```python
from build123d import *

# Parameters (mm, degrees)
BOSS_EXTRUDE1_DEPTH      = 20
SKETCH2_R                = 26.722222222
SKETCH2_R_2              = 17.722222222
BOSS_EXTRUDE2_DEPTH      = 20
CUT_EXTRUDE1_DEPTH       = 65
SKETCH4_R                = 15
BOSS_EXTRUDE3_DEPTH      = 65
CIRPATTERN1_COUNT        = 4
SKETCH5_W                = 98.755733185
SKETCH5_H                = 100
CUT_EXTRUDE2_DEPTH       = 216.315330002
CUT_EXTRUDE2_DEPTH_BACK  = 216.315330002
MOVE_FACE1_BY            = 9
SKETCH6_R                = 26.722222222
SKETCH6_R_2              = 17.722222222
BOSS_EXTRUDE4_DEPTH      = 5
BOSS_EXTRUDE4_DEPTH_BACK = 45


with BuildPart() as part:
    # Sketch1 → Boss-Extrude1 (new, symmetric)
    with BuildSketch(Plane.XY):
        with BuildLine():
            Line((-140.311288741, 0), (-45, 0))
            ThreePointArc((-45, 0), (-43.812144397, 10.271124735), (-40.311288741, 20))
            Line((-40.311288741, 20), (-140.311288741, 20))
            Line((-140.311288741, 20), (-140.311288741, 0))
        make_face()
        with BuildLine():
            ThreePointArc((-40.311288741, -20), (-43.812144397, -10.271124735), (-45, 0))
            Line((-45, 0), (-140.311288741, 0))
            Line((-140.311288741, 0), (-140.311288741, -20))
            Line((-140.311288741, -20), (-40.311288741, -20))
        make_face()
        with BuildLine():
            ThreePointArc((-25, 0), (-17.67766953, 17.67766953), (0, 25))
            Line((0, 25), (9, 25))
            Line((9, 25), (9, 45))
            Line((9, 45), (0, 45))
            ThreePointArc((0, 45), (-23.717082451, 38.242646352), (-40.311288741, 20))
            ThreePointArc((-40.311288741, 20), (-43.812144397, 10.271124735), (-45, 0))
            Line((-45, 0), (-25, 0))
        make_face()
        with BuildLine():
            ThreePointArc((0, -25), (-17.67766953, -17.67766953), (-25, 0))
            Line((-25, 0), (-45, 0))
            ThreePointArc((-45, 0), (-43.812144397, -10.271124735), (-40.311288741, -20))
            ThreePointArc((-40.311288741, -20), (-23.717082451, -38.242646352), (0, -45))
            Line((0, -45), (9, -45))
            Line((9, -45), (9, -25))
            Line((9, -25), (0, -25))
        make_face()
    extrude(amount=BOSS_EXTRUDE1_DEPTH, both=True)

    # Sketch2 → Boss-Extrude2 (add)
    with BuildSketch(Plane(origin=(0, 45, 0), x_dir=(1, 0, 0), z_dir=(0, 1, 0))):
        with Locations((26.722222222, 0)):
            Circle(SKETCH2_R)
        with Locations(Location((26.722222222, 0, 0), (0, 0, 270))):
            Circle(SKETCH2_R_2, mode=Mode.SUBTRACT)
    boss_extrude2 = extrude(amount=-BOSS_EXTRUDE2_DEPTH)

    # Mirror1: Boss-Extrude2 across plane
    add(boss_extrude2.mirror(Plane.ZX))

    # Sketch3 → Cut-Extrude1 (cut)
    with BuildSketch(Plane.ZY.offset(140.311288741)):
        Polygon((-12.5, 20), (-20, 20), (-20, 12.5), align=None)
    cut_extrude1 = extrude(amount=-CUT_EXTRUDE1_DEPTH, mode=Mode.SUBTRACT)

    # Sketch4 → Boss-Extrude3 (add)
    with BuildSketch(Plane.ZY.offset(140.311288741)):
        with Locations(Location((0, 0, 0), (0, 0, 180))):
            Circle(SKETCH4_R)
    extrude(amount=BOSS_EXTRUDE3_DEPTH)

    # CirPattern1: Cut-Extrude1 ×4 about axis
    cirpattern1_axis = Axis((0, 0, 0), (1, 0, 0))
    for i in range(1, CIRPATTERN1_COUNT):
        add(cut_extrude1.rotate(cirpattern1_axis, i * 360 / CIRPATTERN1_COUNT), mode=Mode.SUBTRACT)

    # Sketch5 → Cut-Extrude2 (cut, two sides)
    with BuildSketch(Plane.XY.offset(20)) as cut_extrude2_sk:
        with Locations((9.066577851, 0)):
            Rectangle(SKETCH5_W, SKETCH5_H)
    extrude(amount=CUT_EXTRUDE2_DEPTH, mode=Mode.SUBTRACT)
    extrude(cut_extrude2_sk.sketch, amount=-CUT_EXTRUDE2_DEPTH_BACK, mode=Mode.SUBTRACT)

    # Move Face1: a face moved outward by 9.0
    extrude(part.faces().sort_by_distance((-40.311288741, 0, 0))[0], amount=MOVE_FACE1_BY, dir=(1, 0, 0))

    # Sketch6 → Boss-Extrude4 (add, two sides)
    with BuildSketch(Plane(origin=(0, 20, 0), x_dir=(1, 0, 0), z_dir=(0, 1, 0))) as boss_extrude4_sk:
        with Locations(Location((-13.589066519, 0, 0), (0, 0, 180))):
            Circle(SKETCH6_R)
        with Locations(Location((-13.589066519, 0, 0), (0, 0, 180))):
            Circle(SKETCH6_R_2, mode=Mode.SUBTRACT)
    extrude(amount=BOSS_EXTRUDE4_DEPTH)
    extrude(boss_extrude4_sk.sketch, amount=-BOSS_EXTRUDE4_DEPTH_BACK)


solid = part.part
```
Model file for the job. Use its own axes, mm. A direction names the side the tool comes from. Round coordinates to 2 decimals unless told otherwise and drop trailing zeros. Write each loop counter-clockwise with the first axis right and the second up, starting at its lowest first coordinate (ties: lowest second). Pieces come first, ordered by that corner, then holes. Notation, with made-up numbers: (-12.5, 24) -> (6.5, 24) arc R29 cw to (6.5, 57) -> close; hole circle Ø5 at (55, 4). An arc over 180 degrees is marked (long way). Answer as CSV lines item,"result".
1. Slice it at C-C, the plane x = -26. List the corners of the cut face in (y, z).
Resolved:
outline,"(-25, -23.67) -> (25, -23.67) -> (25, -12.65) -> (-25, -12.65) -> close; (-25, 12.65) -> (25, 12.65) -> (25, 23.67) -> (-25, 23.67) -> close"
2. Slice it at B-B, the plane y = 0. List the corners of the cut face in (x, z), plus the area to 3 significant figures.
Resolved:
outline,"(-205.31, -15) -> (-140.31, -15) -> (-140.31, -20) -> (-31.31, -20) arc R26.72 ccw (long way) to (-31.31, 20) -> (-140.31, 20) -> (-140.31, 15) -> (-205.31, 15) -> close; hole circle Ø35.44 at (-13.59, 0)"
area,"7,320 mm²"
3. Slice it at D-D, the plane x = -97. List the corners of the cut face in (y, z), plus the area to 3 significant figures.
Resolved:
outline,"(-20, -12.5) -> (-12.5, -20) -> (12.5, -20) -> (20, -12.5) -> (20, 12.5) -> (12.5, 20) -> (-12.5, 20) -> (-20, 12.5) -> close"
area,"1,490 mm²"
4. Slice it at A-A, the plane z = 0. List the corners of the cut face in (x, y).
Resolved:
outline,"(-205.31, -15) -> (-140.31, -15) -> (-140.31, -20) -> (-40.31, -20) -> (-40.31, -25) -> (-31.31, -25) -> (-31.31, 25) -> (-40.31, 25) -> (-40.31, 20) -> (-140.31, 20) -> (-140.31, 15) -> (-205.31, 15) -> close; (4.13, -25) -> (13.13, -25) -> (13.13, 25) -> (4.13, 25) -> close"
5. Pin check, flat tips, straight feed: pin 1 Ø12 at (x, z) = (-108, 1) entering from -Y; pin 2 Ø4 at (x, z) = (-93.5, -21.5) entering from -Y; pin 3 Ø10 at (y, z) = (14, -6.5) entering from +X. Stop position of each tip, or through.
Resolved:
pin 1,"y = -20"
pin 2,"y = -13"
pin 3,"x = 13.09"
6. Tool access for faces 1 (the face through (-75.311, 17, 17)), 2 (the face through (-75.311, -17, -17)), 3 (the face through (-108.3, -16.2, 16.3)): list every direction of +Z, -Z, +X, -X, +Y, -Y with a clear straight run to the whole face (end or side of a thin tool).
Resolved:
face 1,"+Z, -X, +Y"
face 2,"-Z, -X, -Y"
face 3,"+Z, -X, -Y"
7. Drill centre lines: line 1 (X direction, y = 15.5, z = -1); line 2 (Z direction, x = -48.5, y = 1.5); line 3 (Z direction, x = -29, y = 1). Where is each one in solid material? Low to high.
Resolved:
line 1,"-140.31 to -31.28, 4.1 to 13.11"
line 2,"-20 to 20"
line 3,"-21.83 to -8.75, 8.75 to 21.83"
